Part model, mm, in its own coordinate system. Face numbers are marked on the shaded views. A direction names the side the tool comes from. Round coordinates to 2 decimals unless told otherwise and drop trailing zeros. Write each loop counter-clockwise with the first axis right and the second up, starting at its lowest first coordinate (ties: lowest second). Pieces come first, ordered by that corner, then holes.
1) Drill centre lines: L1, parallel to Y at x = -93, z = 12.75; L2, parallel to Z at x = -96.25, y = 20; L3, parallel to Y at x = -81, z = 1.5. Where is each one in solid material? Low to high.
2) Saw through at A-A on x = 76. Write the cut outline in (y, z).
3) Pull direction Y, two halves, no side cores. Call the marked faces 1, 2, 3 and 4: +Y half, -Y half, draft (parallel to the pull), parting line (faces both ways), or undercut.
4) Flat gauge pins, fed straight in: pin 1 (12 mm diameter, centred on y = 20, z = 3, fed in from +X); pin 2 (4.5 mm diameter, centred on y = -26.5, z = 11.5, fed in from +X); pin 3 (4 mm diameter, centred on x = 50.5, z = 12.5, fed in from +Y). Where does each tip first touch, or does it go through?
5) Which spindle directions (+Z, -Z, +X, -X, +Y, -Y) get a long thin tool onto all of the face, cutting with end or side? Do the marked faces 5, 6, 7, 8 and 9. Say none if no direction does.
```python
from build123d import *

# Parameters (mm, degrees)
ESBO_O1_R                                           = 17.5
RESSALTO_EXTRUS_O1_DEPTH                            = 25
FILETE1_R                                           = 20
FILETE3_R                                           = 15
CORTE_EXTRUS_O1_DEPTH                               = 156.467038307
ESCAREADO_PARA_PARAFUSO_ALLEN_SEXTAVADO_D           = 17.5
ESCAREADO_PARA_PARAFUSO_ALLEN_SEXTAVADO_CSINK_D     = 33.6
ESCAREADO_PARA_PARAFUSO_ALLEN_SEXTAVADO_CSINK_ANGLE = 90
FURO_ROSCADO_DE_M121_D                              = 10.2
FURO_ROSCADO_DE_M121_DEPTH                          = 25
FURO_ROSCADO_DE_M121_CSINK_D                        = 12.05
FURO_ROSCADO_DE_M121_CSINK_ANGLE                    = 90
FURO_ROSCADO_DE_M121_TIP                            = 3.064389157
FURO_ROSCADO_DE_M122_D                              = 10.2
FURO_ROSCADO_DE_M122_DEPTH                          = 20
FURO_ROSCADO_DE_M122_CSINK_D                        = 12.05
FURO_ROSCADO_DE_M122_CSINK_ANGLE                    = 90
FURO_ROSCADO_DE_M122_TIP                            = 3.064389157
FILETE12_R                                          = 30


with BuildPart() as part:
    # Esboço1 → Ressalto-extrusão1 (new body)
    with BuildSketch(Plane.XY):
        Polygon((-109, 38), (-109, -82), (-29, -82), (-29, -100.739666122), (93, -105), (43, -71.274574158), (43, 20), (21, 42), (9.362419273, 108), (-25.637580727, 108), (-74.652108401, 38), align=None)
        Circle(ESBO_O1_R, mode=Mode.SUBTRACT)
    extrude(amount=RESSALTO_EXTRUS_O1_DEPTH)

    # Filete1
    filete1_edges = [part.edges().sort_by_distance(p)[0] for p in [
        (21, 42, 12.5),
        (43, 20, 12.5),
        (-74.652108401, 38, 12.5),
        (-25.637580727, 108, 12.5),
    ]]
    fillet(filete1_edges, radius=FILETE1_R)

    # Filete3
    filete3_edges = [part.edges().sort_by_distance(p)[0] for p in [
        (9.362419273, 108, 12.5),
    ]]
    fillet(filete3_edges, radius=FILETE3_R)

    # Esboço2 → Corte-extrusão1 (cut, through all)
    with BuildSketch(Plane.XY.offset(25)):
        with BuildLine():
            Line((-20.814924906, 88.735764364), (-54.42488674, 40.735764364))
            ThreePointArc((-54.42488674, 40.735764364), (-55.770535805, 38.007057995), (-56.233366297, 35))
            Line((-56.233366297, 35), (-56.233366297, 31))
            ThreePointArc((-56.233366297, 31), (-53.890220547, 25.343145751), (-48.233366297, 23))
            Line((-48.233366297, 23), (-38.173943993, 23))
            ThreePointArc((-38.173943993, 23), (-31.072198954, 24.303336731), (-24.89605043, 28.043478261))
            ThreePointArc((-24.89605043, 28.043478261), (-14.44771543, 34.605108277), (-2.435454992, 37.420830549))
            ThreePointArc((-2.435454992, 37.420830549), (3.337174211, 40.463464565), (4.9234433, 46.793126488))
            Line((4.9234433, 46.793126488), (-2.05841022, 86.389185421))
            ThreePointArc((-2.05841022, 86.389185421), (-4.794571366, 91.128355545), (-9.936872244, 93))
            Line((-9.936872244, 93), (-12.623404463, 93))
            ThreePointArc((-12.623404463, 93), (-17.240890595, 91.870108332), (-20.814924906, 88.735764364))
        make_face()
        with BuildLine():
            Line((-52.16718427, 3), (-45.224440295, 3))
            ThreePointArc((-45.224440295, 3), (-39.887445215, 0.959570749), (-37.272890353, -4.120879121))
            ThreePointArc((-37.272890353, -4.120879121), (-35.47802498, -12.147417153), (-31.976509443, -19.589610609))
            ThreePointArc((-31.976509443, -19.589610609), (-30.853677224, -24.709534266), (-33.141310542, -29.425581789))
            Line((-33.141310542, -29.425581789), (-43.916738879, -40.201010127))
            ThreePointArc((-43.916738879, -40.201010127), (-47.809819065, -42.802283143), (-52.402020254, -43.715728753))
            Line((-52.402020254, -43.715728753), (-54.357864376, -43.715728753))
            ThreePointArc((-54.357864376, -43.715728753), (-58.1846987, -42.954524078), (-61.428932188, -40.786796564))
            Line((-61.428932188, -40.786796564), (-64.071067812, -38.144660941))
            ThreePointArc((-64.071067812, -38.144660941), (-66.238795325, -34.900427452), (-67, -31.073593129))
            Line((-67, -31.073593129), (-67, -16.370637166))
            ThreePointArc((-67, -16.370637166), (-66.435760282, -13.526287035), (-64.828493161, -11.112703282))
            ThreePointArc((-64.828493161, -11.112703282), (-61.810304111, -7.223226263), (-59.83370305, -2.714285714))
            ThreePointArc((-59.83370305, -2.714285714), (-56.948098707, 1.414269806), (-52.16718427, 3))
        make_face()
        with BuildLine():
            Line((-18.262146843, -38.588048651), (-38.138564286, -58.464466094))
            ThreePointArc((-38.138564286, -58.464466094), (-39.222428043, -63.913417162), (-34.60303038, -67))
            Line((-34.60303038, -67), (-16.5, -67))
            ThreePointArc((-16.5, -67), (-12.964466094, -65.535533906), (-11.5, -62))
            ThreePointArc((-11.5, -62), (-9.613540035, -52.981576235), (-4.270491803, -45.475409836))
            ThreePointArc((-4.270491803, -45.475409836), (-2.861886802, -40.410318309), (-6.762295082, -36.885245902))
            ThreePointArc((-6.762295082, -36.885245902), (-8.184936807, -36.595857818), (-9.595311139, -36.251620711))
            ThreePointArc((-9.595311139, -36.251620711), (-14.240797491, -36.262235776), (-18.262146843, -38.588048651))
        make_face()
    extrude(amount=-CORTE_EXTRUS_O1_DEPTH, mode=Mode.SUBTRACT)

    # Escareado para parafuso Allen sextavado (through all)
    with Locations(Plane(origin=(-79, 3, 25), x_dir=(1, 0, 0), z_dir=(0, 0, 1))):
        with Locations((0, 0), (0, -50), (90, -65)):
            CounterSinkHole(ESCAREADO_PARA_PARAFUSO_ALLEN_SEXTAVADO_D / 2, ESCAREADO_PARA_PARAFUSO_ALLEN_SEXTAVADO_CSINK_D / 2, counter_sink_angle=ESCAREADO_PARA_PARAFUSO_ALLEN_SEXTAVADO_CSINK_ANGLE)

    # Furo roscado de M121
    with Locations(Plane.ZY.offset(109)):
        with Locations((12.5, 20), (12.5, -22), (12.5, -64)):
            CounterSinkHole(FURO_ROSCADO_DE_M121_D / 2, FURO_ROSCADO_DE_M121_CSINK_D / 2, depth=FURO_ROSCADO_DE_M121_DEPTH, counter_sink_angle=FURO_ROSCADO_DE_M121_CSINK_ANGLE)
            with Locations((0, 0, -(FURO_ROSCADO_DE_M121_DEPTH + FURO_ROSCADO_DE_M121_TIP / 2))):  # 118° drill point
                Cone(0, FURO_ROSCADO_DE_M121_D / 2, FURO_ROSCADO_DE_M121_TIP, mode=Mode.SUBTRACT)

    # Furo roscado de M122
    with Locations(Plane(origin=(43, 0, 0), x_dir=(0, 0, -1), z_dir=(1, 0, 0))):
        with Locations((-12.5, -2), (-12.5, -28)):
            CounterSinkHole(FURO_ROSCADO_DE_M122_D / 2, FURO_ROSCADO_DE_M122_CSINK_D / 2, depth=FURO_ROSCADO_DE_M122_DEPTH, counter_sink_angle=FURO_ROSCADO_DE_M122_CSINK_ANGLE)
            with Locations((0, 0, -(FURO_ROSCADO_DE_M122_DEPTH + FURO_ROSCADO_DE_M122_TIP / 2))):  # 118° drill point
                Cone(0, FURO_ROSCADO_DE_M122_D / 2, FURO_ROSCADO_DE_M122_TIP, mode=Mode.SUBTRACT)

    # Filete12
    filete12_edges = [part.edges().sort_by_distance(p)[0] for p in [
        (43, -71.274574158, 12.5),
    ]]
    fillet(filete12_edges, radius=FILETE12_R)


solid = part.part
```
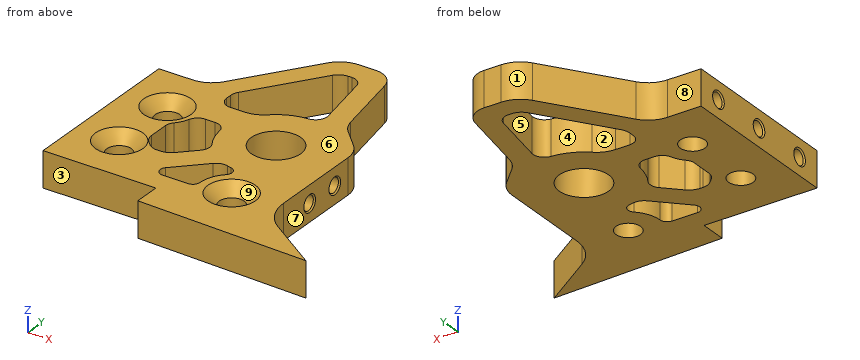
Completed:
1. L1: y = -82 to -69.09, -58.91 to -27.09, -16.91 to 14.91, 25.09 to 38
1. L2: z = 0 to 7.4, 17.6 to 25
1. L3: y = -82 to -55.52, -38.48 to -5.52, 11.52 to 38.42
2. outline: (-104.41, 0) - (-93.53, 0) - (-93.53, 25) - (-104.41, 25) - close
3. face 1: +Y half
3. face 2: undercut
3. face 3: -Y half
3. face 4: undercut
4. pin 1: stops at x = 42.87
4. pin 2: stops at x = 22.37
4. pin 3: stops at y = -72.64
5. face 5: +Z, -Z
5. face 6: +Z, +X, -X, +Y, -Y
5. face 7: +Z, -Z, +X, +Y
5. face 8: +Z, -Z, -X, +Y
5. face 9: +Z
